Here's how the part is built. I have some questions about the finished solid (model axes, mm). A direction names the side the tool comes from. Round coordinates to 2 decimals unless told otherwise and drop trailing zeros. Order: outer loops, then holes, each group sorted by start corner. A loop starts at its lowest first (then second) coordinate and runs counter-clockwise, first axis right, second up. Notation, with made-up numbers: (38, 47.5) -> (72, 47.5) arc R28 cw to (72, 67.5) -> close; hole circle Ø3 at (-27.5, -28). An arc over 180 degrees is marked (long way). One line per item, written item: value.
```python
from build123d import *

# Parameters (mm, degrees)
F0_R            = 26.35
F0_R_2          = 15.7166947943
F1_DEPTH        = 11.3
F2_R            = 17.3887467131
F2_R_2          = 15.7166947943
F3_DEPTH        = 6.4
F4_R            = 24.35
F4_R_2          = 17.3887467131
F5_DEPTH        = 3.3
F6_R            = 3.8017714644
F6_R_2          = 2.75
F7_DEPTH        = 3.4
F7_COPIES_COUNT = 3
F8_DEPTH        = 10
F8_COPIES_COUNT = 3


# Not quite as in the source:
# - a feature of the source that left no trace in its solid (it failed there, or was rolled back) is left out
# - a pattern or mirror of a feature is missing from the dataset's text; its kind, count and spacing are read off the source's solid


with BuildPart() as f1:
    # F0 (on Front) → F1 (new body)
    with BuildSketch(Plane.XZ):
        Circle(F0_R)
        Circle(F0_R_2, mode=Mode.SUBTRACT)
    extrude(amount=F1_DEPTH)

    # F2 (on face) → F3 (cut)
    with BuildSketch(Plane(origin=(0, 0, 0), x_dir=(-1, 0, 0), z_dir=(0, 1, 0))):
        Circle(F2_R)
        Circle(F2_R_2, mode=Mode.SUBTRACT)
    extrude(amount=-F3_DEPTH, mode=Mode.SUBTRACT)

    # F4 (on face) → F5 (cut)
    with BuildSketch(Plane(origin=(0, 0, 0), x_dir=(-1, 0, 0), z_dir=(0, 1, 0))):
        Circle(F4_R)
        Circle(F4_R_2, mode=Mode.SUBTRACT)
    extrude(amount=-F5_DEPTH, mode=Mode.SUBTRACT)

    # F6 (on face) → F7 (cut)
    with BuildSketch(Plane.XZ.offset(11.3)):
        with Locations((0, 21.05)):
            Circle(F6_R)
        with Locations((0, 21.05)):
            Circle(F6_R_2, mode=Mode.SUBTRACT)
    f7 = extrude(amount=-F7_DEPTH, mode=Mode.SUBTRACT)

    # F7_copies: F7 ×3 about axis
    f7_copies_axis = Axis((0, 0, 0), (0, 1, 0))
    for i in range(1, F7_COPIES_COUNT):
        add(f7.rotate(f7_copies_axis, i * 360 / F7_COPIES_COUNT), mode=Mode.SUBTRACT)

    # F8 (cut): a face of the model
    f8_faces = [f1.faces().sort_by_distance(p)[0] for p in [
        (0, -11.3, 21.05),
    ]]
    f8 = extrude(f8_faces, amount=-F8_DEPTH, mode=Mode.SUBTRACT)

    # F8_copies: F8 ×3 about axis
    f8_copies_axis = Axis((0, 0, 0), (0, 1, 0))
    for i in range(1, F8_COPIES_COUNT):
        add(f8.rotate(f8_copies_axis, i * 360 / F8_COPIES_COUNT), mode=Mode.SUBTRACT)


solid = f1.part
```
Q1. I want a section at D-D on z = -22.5. Write out the boundary of the cut face in (x, y).
Answers:
outline: (-13.71, -11.3) -> (13.71, -11.3) -> (13.71, 0) -> (9.31, 0) -> (9.31, -3.3) -> (-9.31, -3.3) -> (-9.31, 0) -> (-13.71, 0) -> close
Q2. I want a section at C-C on x = -18.5. Write out the boundary of the cut face in (y, z), then the cut area to 3 significant figures.
Answers:
outline: (-11.3, -18.76) -> (0, -18.76) -> (0, -15.83) -> (-3.3, -15.83) -> (-3.3, -13.26) -> (-7.9, -13.26) -> (-7.9, -14.32) -> (-11.3, -14.32) -> close; (-11.3, -6.73) -> (-7.9, -6.73) -> (-7.9, -7.79) -> (-3.3, -7.79) -> (-3.3, 15.83) -> (0, 15.83) -> (0, 18.76) -> (-11.3, 18.76) -> close
area: 269 mm2
Q3. Which directions (+Z, -Z, +X, -X, +Y, -Y) give clear straight access to the entire face, cutting with the end or side of a thin tool? Please do faces 1 (the face through (11.3, -11.3, -11.3)), 2 (the face through (19.32, -1.63, -14.82)), 3 (the face through (3, -7.9, 22)).
Answers:
face 1: +Z, -Z, +X, -X, -Y
face 2: +Y
face 3: -Y
Q4. For P1, Ø7, axis at x = -18.23, z = -10.53, coming from the +Y side; P2, Ø6, axis at x = 11.5, y = -5.5, coming from the -Z side; P3, Ø1.5, axis at y = -6, z = 5, coming from the +X side (3 decimals); P4, Ø2, axis at y = -9.5, z = -2.5, coming from the -X side, each with a flat end and sliding along its axis, tell me the tip position at first contact or that it passes through.
Answers:
P1: y = 0
P2: z = -24.94
P3: x = 26.005
P4: x = -26.31
Q5. I want a section at B-B on x = 0. Write out the boundary of the cut face in (y, z).
Answers:
outline: (-11.3, -26.35) -> (0, -26.35) -> (0, -24.35) -> (-3.3, -24.35) -> (-3.3, -17.39) -> (-6.4, -17.39) -> (-6.4, -15.72) -> (-11.3, -15.72) -> close; (-11.3, 15.72) -> (-6.4, 15.72) -> (-6.4, 17.39) -> (-3.3, 17.39) -> (-3.3, 18.3) -> (-7.9, 18.3) -> (-7.9, 17.25) -> (-11.3, 17.25) -> close; (-11.3, 24.85) -> (-7.9, 24.85) -> (-7.9, 23.8) -> (-3.3, 23.8) -> (-3.3, 24.35) -> (0, 24.35) -> (0, 26.35) -> (-11.3, 26.35) -> close
Q6. If we mould it in two halves opening along X, with no side actions, what happens to faces 4 (the face through (-5.712, -5.571, -25.723)), 5 (the face through (15.482, -5.632, -10.404)), 6 (the face through (7.7, 0, -23.3))? For each: pulls with the +X half, pulls with the -X half, needs draft (parallel to the pull), parting line crosses it, or undercut.
Answers:
face 4: parting line crosses it
face 5: undercut
face 6: needs draft
Q7. I want a section at A-A on z = 0. Write out the boundary of the cut face in (x, y), then the cut area to 3 significant figures.
Answers:
outline: (-26.35, -11.3) -> (-15.72, -11.3) -> (-15.72, -6.4) -> (-17.39, -6.4) -> (-17.39, -3.3) -> (-24.35, -3.3) -> (-24.35, 0) -> (-26.35, 0) -> close; (15.72, -11.3) -> (26.35, -11.3) -> (26.35, 0) -> (24.35, 0) -> (24.35, -3.3) -> (17.39, -3.3) -> (17.39, -6.4) -> (15.72, -6.4) -> close
area: 173 mm2
Q8. I need wall thicknesses on line 1 along Z through (x, y) = (0, -4.8); line 2 along X through (y, z) = (-2, -0.5); line 3 along Z through (x, y) = (-0.5, -6.5). Which ranges of each line are inside material? Lowest first, please.
Answers:
line 1: -26.35 to -17.39, 17.39 to 18.3, 23.8 to 26.35
line 2: -26.35 to -24.34, 24.34 to 26.35
line 3: -26.35 to -15.71, 15.71 to 18.35, 23.75 to 26.35
